```python
from build123d import *

# Parameters (mm, degrees)
SKETCH1_R           = 1.321708294
SKETCH2_R           = 0.804719078
SKETCH5_R           = 0.804719078
BOSS_EXTRUDE2_DEPTH = 0.1
SKETCH6_R           = 0.804719078
SKETCH7_R           = 0.987442809
SKETCH8_W           = 1.974885617
SKETCH8_H           = 1.974885617
BOSS_EXTRUDE3_DEPTH = 0.3125


with BuildPart() as part:
    # Sketch1 → Loft1 section 0
    with BuildSketch(Plane.XY):
        with Locations((7.853314297, -30.890436458)):
            Circle(SKETCH1_R)
    # Sketch2 → Loft1 section 1
    with BuildSketch(Plane.XY.offset(10)):
        with Locations((7.853314297, -30.890436458)):
            Circle(SKETCH2_R)
    loft()

    # Sketch5 → Boss-Extrude2 (add)
    with BuildSketch(Plane.XY.offset(10)):
        with Locations((7.853314297, -30.890436458)):
            Circle(SKETCH5_R)
    extrude(amount=BOSS_EXTRUDE2_DEPTH)

    # Sketch6 → Loft2 section 0
    with BuildSketch(Plane.XY.offset(10.1)):
        with Locations((7.853314297, -30.890436458)):
            Circle(SKETCH6_R)
    # Sketch7 → Loft2 section 1
    with BuildSketch(Plane.XY.offset(10.3125)):
        with Locations((7.853314297, -30.890436458)):
            Circle(SKETCH7_R)
    loft()

    # Sketch8 → Boss-Extrude3 (add)
    with BuildSketch(Plane.XY.offset(10.3125)):
        with Locations((7.853314298, -30.890436459)):
            Rectangle(SKETCH8_W, SKETCH8_H)
    extrude(amount=BOSS_EXTRUDE3_DEPTH)


solid = part.part
```
Can you work these out from the model? Positions are in its coordinate system, mm. Coordinates: 2 decimals unless noted, no trailing zeros. Loops run counter-clockwise (first coordinate to the right, second up) from the corner with the lowest first, then second, coordinate; pieces in that order, holes last. Notation, with made-up numbers: (27.5, 4.25) - (53.5, 4.25) arc R21 ccw to (53.5, 41.25) - close; hole circle Ø6 at (87.25, -30). An arc over 180 degrees is marked (long way). Answer as CSV lines item,"result". Start each with the question number.
1) Thinking about a two-plate mould opening in Z: for faces 1 (the flat face through (8, -31, 10.625)), 2 (the conical face through (7.624, -31.925, 5.07)), 3 (the flat face through (8, -31, 0)), which applies, pulls with the +Z half, pulls with the -Z half, needs draft (parallel to the pull), parting line crosses it, or undercut?
2) For pin 1 (1.5 mm diameter, centred on x = 8.5, z = 2, fed in from +Y); pin 2 (1 mm diameter, centred on x = 7.5, z = 9.5, fed in from -Y), each with a flat end and sliding along its axis, tell me the tip position at first contact or that it passes through.
3) I need wall thicknesses on line 1 (X direction, y = -31.6, z = 6.25); line 2 (Y direction, x = 7.3, z = 2.25); line 3 (X direction, y = -31.3, z = 8). Which ranges of each line are inside material? Lowest first, please. Write a range as from..to.
4) Suppose I cut it at B-B (z = 9.5). Please give me the cut outline in (x, y), plus the area to 3 significant figures.
5) Suppose I cut it at A-A (z = 4.5). Please give me the cut outline in (x, y).
Check result:
1,face 1,"pulls with the +Z half"
1,face 2,"undercut"
1,face 3,"pulls with the -Z half"
2,pin 1,"stops at y = -29.65"
2,pin 2,"stops at y = -31.74"
3,line 1,"x = 7.15..8.56"
3,line 2,"y = -31.96..-29.82"
3,line 3,"x = 7.04..8.66"
4,outline,"circle Ø1.66 at (7.85, -30.89)"
4,area,"2.17 mm²"
5,outline,"circle Ø2.18 at (7.85, -30.89)"
